Input: part model. Units: mm. Frame: model coordinates. Face numbers are marked on the shaded views. Coordinates: 2 decimals unless noted, no trailing zeros. Order: outer loops, then holes, each group sorted by start corner. A loop starts at its lowest first (then second) coordinate and runs counter-clockwise, first axis right, second up. Notation, with made-up numbers: (33.5, -19) - (77.5, -19) arc R23 ccw to (77.5, 9) - close; hole circle Ø6 at (-13, -3). An arc over 180 degrees is marked (long way). Answer as CSV lines item,"result". Start each with the question number.
Item 1: Section C-C (z = 2.15). State how many separate pieces and enclosed holes the cut face has, and give its area (3 significant figures).
Item 2: Section B-B (x = 34). Output: boundary loops of the cut face in (y, z) (3 decimals).
Item 3: Section D-D (y = -39). Output: boundary loops of the cut face in (x, z) (1 decimal), and give its area (3 significant figures).
Item 4: Material intervals for line 1 along Y through (x, z) = (2.54, 2.4); line 2 along Y through (x, z) = (2, 2.5); line 3 along X through (y, z) = (-39, 0.4), sorted ascending.
Item 5: Section A-A (y = -25.4). Output: boundary loops of the cut face in (x, z) (1 decimal).
Item 6: Draft query along Z for the marked faces 1 and 2. Return one class per face: +Z half, -Z half, draft (parallel to the pull), parting line (faces both ways), or undercut.
from build123d import *

# Parameters (mm, degrees)
F0_R     = 1.143
F0_R_2   = 1.2065
F0_R_3   = 9.525
F1_DEPTH = 3.175


with BuildPart() as f1:
    # F0 (on Top) → F1 (new body)
    with BuildSketch(Plane.XY):
        with BuildLine():
            Line((52.451, 0), (2.54, 0))
            ThreePointArc((2.54, 0), (0.743949, -0.743949), (0, -2.54))
            Line((0, -2.54), (0, -62.559217))
            Line((0, -62.559217), (17.044382, -62.559217))
            Line((17.044382, -62.559217), (17.044382, -68.58))
            Line((17.044382, -68.58), (54.991, -68.58))
            Line((54.991, -68.58), (54.991, -55.58028))
            Line((54.991, -55.58028), (46.9265, -55.58028))
            Line((46.9265, -55.58028), (46.9265, -4.582543))
            Line((46.9265, -4.582543), (54.991, -4.582543))
            Line((54.991, -4.582543), (54.991, -2.54))
            ThreePointArc((54.991, -2.54), (54.247051, -0.743949), (52.451, 0))
        make_face()
        with Locations((2.54, -60.019217)):
            Circle(F0_R, mode=Mode.SUBTRACT)
        with Locations((52.451, -58.12028)):
            Circle(F0_R, mode=Mode.SUBTRACT)
        with Locations((37.8968, -35.93797)):
            Circle(F0_R_2, mode=Mode.SUBTRACT)
        with Locations((2.54, -2.54)):
            Circle(F0_R, mode=Mode.SUBTRACT)
        with Locations((17.860312, -14.858122)):
            Circle(F0_R_2, mode=Mode.SUBTRACT)
        with Locations((27.8765, -25.4)):
            Circle(F0_R_3, mode=Mode.SUBTRACT)
        with Locations((37.892688, -14.858122)):
            Circle(F0_R_2, mode=Mode.SUBTRACT)
        with Locations((52.451, -2.54)):
            Circle(F0_R, mode=Mode.SUBTRACT)
    extrude(amount=F1_DEPTH)


solid = f1.part
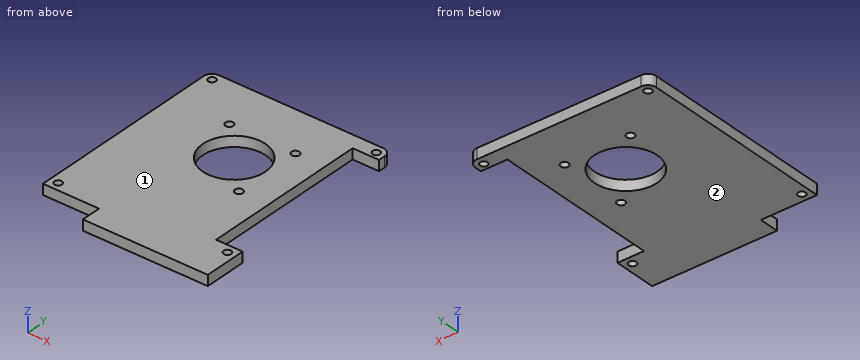
Determined:
1,separate pieces,"1"
1,enclosed holes,"8"
1,area,"2,940 mm^2"
2,outline,"(-68.58, 0) - (-32.696, 0) - (-32.696, 3.175) - (-68.58, 3.175) - close; (-18.104, 0) - (0, 0) - (0, 3.175) - (-18.104, 3.175) - close"
3,outline,"(0, 0) - (46.9, 0) - (46.9, 3.2) - (0, 3.2) - close"
3,area,"149 mm^2"
4,line 1,"y = -62.56 to -61.16, -58.88 to -3.68, -1.4 to 0"
4,line 2,"y = -62.56 to -61.03, -59.01 to -3.55, -1.53 to -0.06"
4,line 3,"x = 0 to 46.93"
5,outline,"(0, 0) - (18.4, 0) - (18.4, 3.2) - (0, 3.2) - close; (37.4, 0) - (46.9, 0) - (46.9, 3.2) - (37.4, 3.2) - close"
6,face 1,"+Z half"
6,face 2,"-Z half"
